Source: CAD feature listing. Evaluate the final solid. Frame: model axes, mm. A direction names the side the tool comes from. Round coordinates to 2 decimals unless told otherwise and drop trailing zeros. Loops run counter-clockwise (first coordinate to the right, second up) from the corner with the lowest first, then second, coordinate; pieces in that order, holes last. Notation, with made-up numbers: M 71,17 L 82,17 A15 cw 82,26 Z; hole C 10,-20.5 d3. An arc over 180 degrees is marked long. One line per item, written item: value.
from build123d import *

# Parameters (mm, degrees)
SKETCH_1_W             = 64
SKETCH_1_H             = 52
EXTRUDE_348_DEPTH      = 8
EXTRUDE_START          = -40
SKETCH_2_W             = 104
SKETCH_2_H             = 6
EXTRUDE_C_6_DEPTH      = 41
SKETCH_3_W             = 104
SKETCH_3_H             = 6
EXTRUDE_C_6_2_DEPTH    = 41
EXTRUDE_START_2        = -32
EXTRUDE_798_DEPTH      = 6
EXTRUDE_START_3        = 26
EXTRUDE_5_DEPTH        = 6
CUT_EXTRUDE_8_DEPTH    = 8
CUT_EXTRUDE_START      = -11.5
SKETCH_7_R             = 2.5
CUT_EXTRUDE_1237_DEPTH = 18


with BuildPart() as part:
    # 草图1 → Extrude 348 (new body)
    with BuildSketch(Plane.XY):
        with Locations((0, 14.5)):
            Rectangle(SKETCH_1_W, SKETCH_1_H)
    extrude(amount=EXTRUDE_348_DEPTH)

    # 草图2 → Extrude C_6 (add)
    with BuildSketch(Plane.XY.offset(EXTRUDE_START)):
        with Locations((0, -8.5)):
            Rectangle(SKETCH_2_W, SKETCH_2_H)
    extrude(amount=EXTRUDE_C_6_DEPTH)

    # 草图3 → Extrude C_6 2 (add)
    with BuildSketch(Plane.XY.offset(EXTRUDE_START)):
        with Locations((0, 3.5)):
            Rectangle(SKETCH_3_W, SKETCH_3_H)
    extrude(amount=EXTRUDE_C_6_2_DEPTH)

    # 草图4 → Extrude 798 (add)
    with BuildSketch(Plane(origin=(0, 0, 0), x_dir=(0, 0, -1), z_dir=(1, 0, 0)).offset(EXTRUDE_START_2)):
        Polygon((28, 6.5), (-1, 6.5), (-1, 38.5), align=None)
    extrude(amount=EXTRUDE_798_DEPTH)

    # 草图5 → 凸台-拉伸5 (add)
    with BuildSketch(Plane(origin=(0, 0, 0), x_dir=(0, 0, -1), z_dir=(1, 0, 0)).offset(EXTRUDE_START_3)):
        Polygon((28, 6.5), (-1, 6.5), (-1, 38.5), align=None)
    extrude(amount=EXTRUDE_5_DEPTH)

    # 草图6 → 上下可调槽_中心行程正负8 (cut)
    with BuildSketch(Plane.XY):
        with BuildLine():
            Line((-8, 14.5), (-8, 30.5))
            ThreePointArc((-8, 30.5), (-10, 32.5), (-12, 30.5))
            Line((-12, 30.5), (-12, 14.5))
            ThreePointArc((-12, 14.5), (-10, 12.5), (-8, 14.5))
        make_face()
        with BuildLine():
            Line((12, 14.5), (12, 30.5))
            ThreePointArc((12, 30.5), (10, 32.5), (8, 30.5))
            Line((8, 30.5), (8, 14.5))
            ThreePointArc((8, 14.5), (10, 12.5), (12, 14.5))
        make_face()
    extrude(amount=CUT_EXTRUDE_8_DEPTH, mode=Mode.SUBTRACT)

    # 草图7 → Cut-Extrude 1237 (cut)
    with BuildSketch(Plane(origin=(0, 0, 0), x_dir=(1, 0, 0), z_dir=(0, 1, 0)).offset(CUT_EXTRUDE_START)):
        with Locations(Location((-42, 30, 0), (0, 0, 270))):
            Circle(SKETCH_7_R)
        with Locations(Location((42, 30, 0), (0, 0, 270))):
            Circle(SKETCH_7_R)
    extrude(amount=CUT_EXTRUDE_1237_DEPTH, mode=Mode.SUBTRACT)


solid = part.part
1. Section query B-B (x = -38). Return the cut outline in (y, z).
Report:
outline: M -11.5,-40 L -5.5,-40 L -5.5,1 L -11.5,1 Z; M 0.5,-40 L 6.5,-40 L 6.5,1 L 0.5,1 Z
2. Section query A-A (z = -36). Return the cut outline in (x, y).
Report:
outline: M -52,-11.5 L 52,-11.5 L 52,-5.5 L -52,-5.5 Z; M -52,0.5 L 52,0.5 L 52,6.5 L -52,6.5 Z
3. Ray query, line 1 (Z direction, x = -42, y = 4.4); line 2 (Y direction, x = -10, z = 0.5); line 3 (Y direction, x = -42, z = -13). Return the intervals inside material, ascending. Write a range as [from, to].
Report:
line 1: z = [-40, -32.5], [-27.5, 1]
line 2: y = [-11.5, 12.5], [32.5, 40.5]
line 3: y = [-11.5, -5.5], [0.5, 6.5]
4. Pull-direction query (Z, two-part tool) for faces 1 (the face through (28.958, 22.165, -13.804)), 2 (the face through (39.56, -8.54, -30.54)), 3 (the face through (-1, -5.5, -20)); classes: released by +Z, released by -Z, zero draft, split by the parting line, or undercut.
Report:
face 1: released by -Z
face 2: undercut
face 3: zero draft
5. Reachability of faces 4 (the face through (42, -8, 1)), 5 (the face through (-1, 6.5, -20)), 6 (the face through (8, 23, 4)) from +Z, -Z, +X, -X, +Y, -Y: full face, straight path, thin tool, end or side. Return the list, or none.
Report:
face 4: +Z, +X, +Y, -Y
face 5: -Z, +Y
face 6: +Z, -Z
6. Section query C-C (y = 19). Return the cut outline in (x, z).
Report:
outline: M -32,-16.67 L -26,-16.67 L -26,0 L -12,0 L -12,8 L -32,8 Z; M -8,0 L 8,0 L 8,8 L -8,8 Z; M 12,0 L 26,0 L 26,-16.67 L 32,-16.67 L 32,8 L 12,8 Z
7. Section query D-D (z = -30). Return the cut outline in (x, y).
Report:
outline: M -52,-11.5 L -44.5,-11.5 L -44.5,-5.5 L -52,-5.5 Z; M -52,0.5 L -44.5,0.5 L -44.5,6.5 L -52,6.5 Z; M -39.5,-11.5 L 39.5,-11.5 L 39.5,-5.5 L -39.5,-5.5 Z; M -39.5,0.5 L 39.5,0.5 L 39.5,6.5 L -39.5,6.5 Z; M 44.5,-11.5 L 52,-11.5 L 52,-5.5 L 44.5,-5.5 Z; M 44.5,0.5 L 52,0.5 L 52,6.5 L 44.5,6.5 Z
8. Pin query (flat end, axial travel): pin 1 (20.5 mm diameter, centred on x = 9, z = -22.5, fed in from +Y); pin 2 (3 mm diameter, centred on x = -45.5, y = 2.5, fed in from +Z); pin 3 (9 mm diameter, centred on y = 23.5, z = 3.5, fed in from +X). Return the tip coordinate at first contact, or that it passes through.
Report:
pin 1: stops at y = 6.5
pin 2: stops at z = 1
pin 3: stops at x = 32
